Autodesk Inventor part; units mm, degrees
ref_plane "YZ Plane" through (0, 0, 0) normal (1, 0, 0) x (0, 1, 0)
ref_plane "XZ Plane" through (0, 0, 0) normal (0, 1, 0) x (-1, 0, 0)
ref_plane "XY Plane" through (0, 0, 0) normal (0, 0, 1) x (1, 0, 0)
sketch "Sketch1" plane through (0, 0, 0) normal (0, 1, 0) x (-1, 0, 0)
  circle A0 centre (0, 0) radius 39.5
  circle A1 centre (0, 0) radius 31.5
  circle A2 centre (0, 0) radius 28
  line L0 (-28.5, 13.4164) -> (-28.5, -13.4164)
  circle A3 centre (0, 0) radius 36 construction
  line L1 (0, 39.5) -> (0, 0) construction
  line L2 (0, 0) -> (-34.208, 19.75) construction
  circle A4 centre (0, 36) radius 1.4
  circle A5 centre (-31.1769, 18) radius 1.4
  line L3 (0, 0) -> (-39.5, 0) construction
  circle A6 centre (31.1769, 18) radius 1.4
  circle A7 centre (0, -36) radius 1.4
  circle A8 centre (-31.1769, -18) radius 1.4
  circle A9 centre (31.1769, -18) radius 1.4
  circle A10 centre (0, 0) radius 22.5
  dimension "d0" = 79
  dimension "d1" = 63
  dimension "d2" = 56
  dimension "d6" = 28.5
  dimension "d11" = 72
  dimension "d12" = 2.8
  dimension "d13" = 60
  dimension "d19" = 45
extrude "Extrusion1" add sketch "Sketch1" along normal blind 29 contours A0 | A1 L0 | L0 A1 | A2 | A4 | A5 | A6 | A7 | A8 | A9 | A10
extrude "Extrusion2" add sketch "Sketch1" against normal blind 11.5 contours A1 L0 | A2 | A10 picked at (29.747, 4.7866)
extrude "Extrusion3" add sketch "Sketch1" along normal blind 2.5 from surface at 29 contours A2 | A10
extrude "Extrusion4" cut sketch "Sketch1" along normal blind 15 contours A4 | A5 | A6 | A7 | A8 | A9
chamfer "Chamfer1" distance 1 angle 45 6 edges at (1.4, 0, -36) (-29.7769, 0, -18) (-29.7769, 0, 18) (32.5769, 0, -18) (32.5769, 0, 18) (1.4, 0, 36)
extrude "Extrusion5" cut sketch "Sketch1" along normal blind 29 and the other way blind 8.25 contours A10
fillet "Fillet1" radius 1 1 edges at (39.5, 0, 0)
fillet "Fillet2" radius 1 1 edges at (39.5, 29, 0)
properties part number "motor_simplified"
Source: CAD feature listing. Evaluate the final solid. Frame: model axes, mm. A direction names the side the tool comes from. Give positions to 0.01 mm unless a question says otherwise; leave off trailing zeros. Loops run counter-clockwise (first coordinate to the right, second up) from the corner with the lowest first, then second, coordinate; pieces in that order, holes last. Notation, with made-up numbers: M 23,34 L 32,34 A25 ccw 32,46 Z; hole C 79.25,30.5 d11. An arc over 180 degrees is marked long. Put each result on its own line as item: value.
Q1. Mould query, pull axis Y, two halves, no side actions, for faces 1 (the flat face through (0, 31.5, 0)), 2 (the flat face through (0, 15, -36)), 3 (the flat face through (0, 29, 0)), 4 (the cylindrical face through (0.18, 7.9, 34.61)). Classes: released by +Y, released by -Y, zero draft, split by the parting line, or undercut.
Response values:
face 1: released by +Y
face 2: released by -Y
face 3: undercut
face 4: zero draft
Q2. Section C-C (y = 9). Return the cut outline in (x, z), and give its area (3 significant figures).
Response values:
outline: C 0,0 d79; hole C -31.18,-18 d2.8; hole C -31.18,18 d2.8; hole C 0,0 d45; hole C 0,-36 d2.8; hole C 0,36 d2.8; hole C 31.18,-18 d2.8; hole C 31.18,18 d2.8
area: 3,270 mm²
Q3. Section D-D (y = 23). Return the cut outline in (x, z), and give its area (3 significant figures).
Response values:
outline: C 0,0 d79; hole C 0,0 d45
area: 3,310 mm²
Q4. Pin query (flat end, axial travel): P1, Ø1.4, axis at x = 0, z = 36.5, coming from the -Y side; P2, Ø3, axis at x = -17, y = 20, coming from the +Z side; P3, Ø4, axis at y = 13, z = 22.5, coming from the -X side. Return the tip coordinate at first contact, or that it passes through.
Response values:
P1: stops at y = 15
P2: stops at z = 36.33
P3: stops at x = -33.76
Q5. Reachability of faces 5 (the flat face through (-1, -11.5, 0)), 6 (the cylindrical face through (-10.382, 10.114, 19.961)), 7 (the flat face through (31, 15, 18)), 8 (the cylindrical face through (-25.865, 30.232, 10.724)) from +Z, -Z, +X, -X, +Y, -Y: full face, straight path, thin tool, end or side. Return the list, or none.
Response values:
face 5: +Z, -Z, +X, -X, -Y
face 6: none
face 7: -Y
face 8: +Y
Q6. Line query: probe 1 along Z at (x, y) = (0, 5.5); probe 2 along Y at (x, z) = (14.5, -1); probe 3 along Y at (x, z) = (-30.5, 19). Output: solid intervals per line, ascending. Write a range as [from, to].
Response values:
probe 1: z = [-39.5, -37.4], [-34.6, -22.5], [22.5, 34.6], [37.4, 39.5]
probe 2: y = [-11.5, -8.25], [29, 31.5]
probe 3: y = [15, 29]
Q7. Section A-A (z = 0). Return the cut outline in (x, y).
Response values:
outline: M -39.5,1 A1 ccw -38.5,0 L -31.5,0 L -31.5,-11.5 L 28.5,-11.5 L 28.5,0 L 38.5,0 A1 ccw 39.5,1 L 39.5,28 A1 ccw 38.5,29 L 28,29 L 28,31.5 L -28,31.5 L -28,29 L -38.5,29 A1 ccw -39.5,28 Z; hole M -22.5,-8.25 L 22.5,-8.25 L 22.5,29 L -22.5,29 Z
